Geometry check sheet. Reference: drawing and pictorial views, mm from the part's lowest x, y, z. A direction names the side the tool comes from. Round coordinates to 2 decimals unless told otherwise and drop trailing zeros. Order: outer loops, then holes, each group sorted by start corner. A loop starts at its lowest first (then second) coordinate and runs counter-clockwise, first axis right, second up.
(1) Set-up check for the marked faces 1 and 2: record each of +Z, -Z, +X, -X, +Y, -Y from which the full face is reachable in a straight line by a thin tool's end or side.
(2) Release check for a two-part mould opening along Y. For the marked faces 3, 4 and 5 record: +Y half, -Y half, draft (parallel to the pull), parting line (faces both ways), or undercut.
(3) Sectioned sample at C-C (z = 3.4). Record the boundary of the cut face in (x, y), plus the area to 3 significant figures.
(4) Go/stop test with flat-tipped pins: pin 1 (2 mm diameter, centred on y = 8, z = 2.5, fed in from +X); pin 2 (2.5 mm diameter, centred on x = 4.5, y = 3, fed in from +Z); pin 3 (1.5 mm diameter, centred on y = 2.5, z = 3.5, fed in from -X); pin 4 (3 mm diameter, centred on x = 5, y = 5, fed in from -Z). Record where each tip stops, or that it passes through.
(5) Material ranges on line 1 along Y through (x, z) = (5, 2.35) (3 decimals); line 2 along Y through (x, z) = (6, 2.95); line 3 along Y through (x, z) = (5, 1.45) (3 decimals), recorded low to high.
(6) Sectioned sample at A-A (y = 5). Record the boundary of the cut face in (x, z) (3 decimals).
(7) Sectioned sample at D-D (x = 1.5). Record the boundary of the cut face in (y, z).
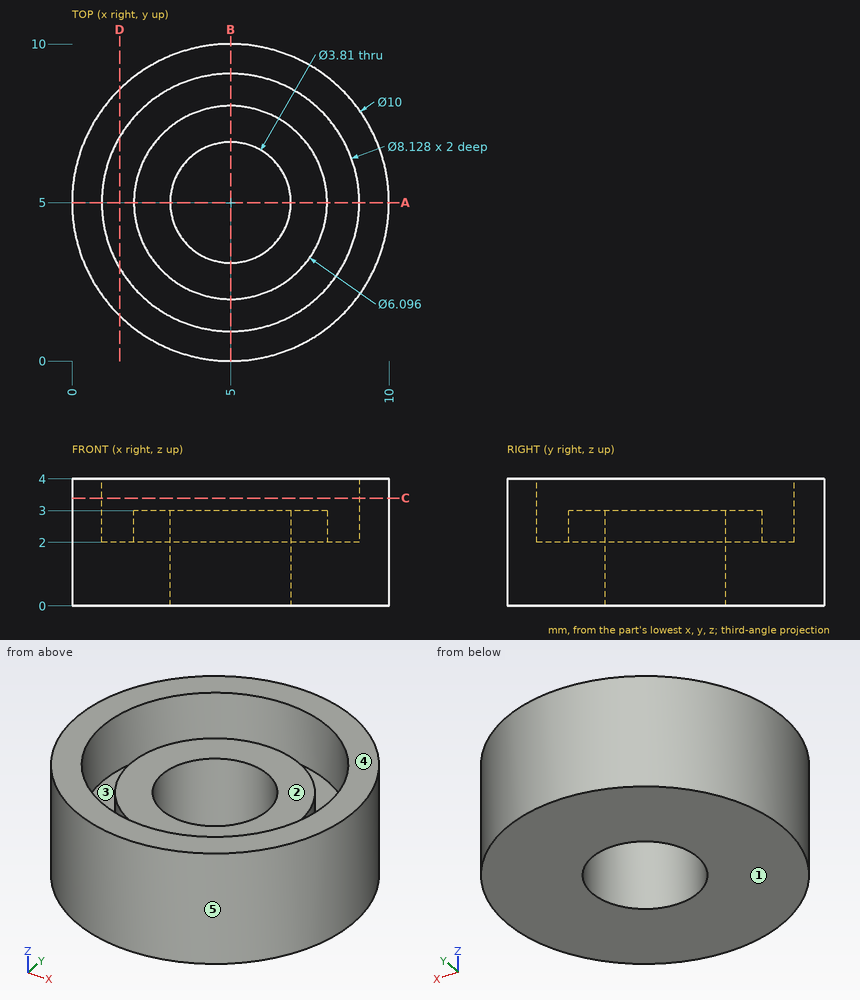
Answer below:
1. face 1: -Z, +X, -X, +Y, -Y
1. face 2: +Z
2. face 3: undercut
2. face 4: draft
2. face 5: parting line
3. outline: circle Ø10 at (5, 5); hole circle Ø8.13 at (5, 5)
3. area: 26.7 mm2
4. pin 1: stops at x = 9.58
4. pin 2: stops at z = 3
4. pin 3: stops at x = 0.32
4. pin 4: passes through
5. line 1: y = 0 to 0.936, 1.952 to 3.095, 6.905 to 8.048, 9.064 to 10
5. line 2: y = 0.1 to 1.06, 2.12 to 3.38, 6.62 to 7.88, 8.94 to 9.9
5. line 3: y = 0 to 3.095, 6.905 to 10
6. outline: (0, 0) - (3.095, 0) - (3.095, 3) - (1.952, 3) - (1.952, 2) - (0.936, 2) - (0.936, 4) - (0, 4) - close; (6.905, 0) - (10, 0) - (10, 4) - (9.064, 4) - (9.064, 2) - (8.048, 2) - (8.048, 3) - (6.905, 3) - close
7. outline: (1.43, 0) - (8.57, 0) - (8.57, 4) - (7.07, 4) - (7.07, 2) - (2.93, 2) - (2.93, 4) - (1.43, 4) - close
